The model under review builds one solid part; all positions refer to its coordinate system, in mm. Face numbers are marked on the shaded views. A direction names the side the tool comes from. Coordinates: 2 decimals unless noted, no trailing zeros. Order: outer loops, then holes, each group sorted by start corner. A loop starts at its lowest first (then second) coordinate and runs counter-clockwise, first axis right, second up.
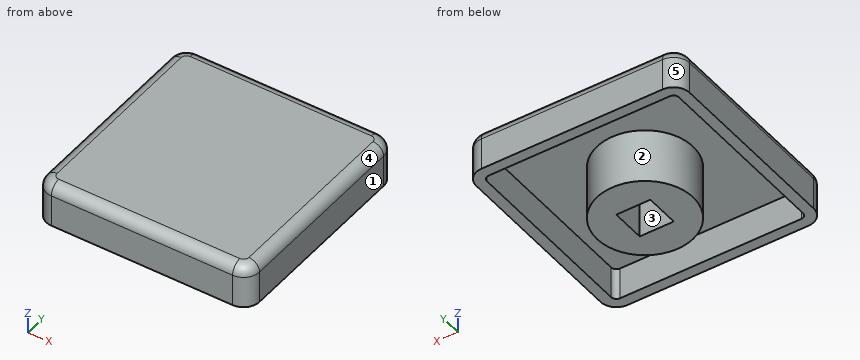
```python
from build123d import *

# Parameters (mm, degrees)
SKETCH1_R           = 4.5
SKETCH1_W           = 3.2
SKETCH1_H           = 3.2
BOSS_EXTRUDE1_DEPTH = 5.1
BOSS_EXTRUDE2_DEPTH = 1
BOSS_EXTRUDE3_START = 3
BOSS_EXTRUDE3_DEPTH = 3
FILLET1_R           = 1


with BuildPart() as part:
    # Sketch1 → Boss-Extrude1 (new body)
    with BuildSketch(Plane.XY):
        Circle(SKETCH1_R)
        Rectangle(SKETCH1_W, SKETCH1_H, mode=Mode.SUBTRACT)
    extrude(amount=BOSS_EXTRUDE1_DEPTH)

    # Sketch2 → Boss-Extrude2 (add)
    with BuildSketch(Plane.XY.offset(5.1)):
        with BuildLine():
            Line((-8.5, -10), (8.5, -10))
            ThreePointArc((8.5, -10), (9.560660172, -9.560660172), (10, -8.5))
            Line((10, -8.5), (10, 8.5))
            ThreePointArc((10, 8.5), (9.560660172, 9.560660172), (8.5, 10))
            Line((8.5, 10), (-8.5, 10))
            ThreePointArc((-8.5, 10), (-9.560660172, 9.560660172), (-10, 8.5))
            Line((-10, 8.5), (-10, -8.5))
            ThreePointArc((-10, -8.5), (-9.560660172, -9.560660172), (-8.5, -10))
        make_face()
    extrude(amount=BOSS_EXTRUDE2_DEPTH)

    # Sketch3 → Boss-Extrude3 (add)
    with BuildSketch(Plane(origin=(0, 0, 5.1), x_dir=(-1, 0, 0), z_dir=(0, 0, -1)).offset(BOSS_EXTRUDE3_START)):
        with BuildLine():
            Line((-8.5, -10), (8.5, -10))
            ThreePointArc((8.5, -10), (9.560660172, -9.560660172), (10, -8.5))
            Line((10, -8.5), (10, 8.5))
            ThreePointArc((10, 8.5), (9.560660172, 9.560660172), (8.5, 10))
            Line((8.5, 10), (-8.5, 10))
            ThreePointArc((-8.5, 10), (-9.560660172, 9.560660172), (-10, 8.5))
            Line((-10, 8.5), (-10, -8.5))
            ThreePointArc((-10, -8.5), (-9.560660172, -9.560660172), (-8.5, -10))
        make_face()
        with BuildLine():
            Line((8.5, 9), (-8.5, 9))
            ThreePointArc((-8.5, 9), (-8.853553391, 8.853553391), (-9, 8.5))
            Line((-9, 8.5), (-9, -8.5))
            ThreePointArc((-9, -8.5), (-8.853553391, -8.853553391), (-8.5, -9))
            Line((-8.5, -9), (8.5, -9))
            ThreePointArc((8.5, -9), (8.853553391, -8.853553391), (9, -8.5))
            Line((9, -8.5), (9, 8.5))
            ThreePointArc((9, 8.5), (8.853553391, 8.853553391), (8.5, 9))
        make_face(mode=Mode.SUBTRACT)
    extrude(amount=-BOSS_EXTRUDE3_DEPTH)

    # Fillet1
    fillet1_edges = [part.edges().sort_by_distance(p)[0] for p in [
        (9.560660172, -9.560660172, 6.1),
        (10, 0, 6.1),
        (9.560660172, 9.560660172, 6.1),
        (0, 10, 6.1),
        (-9.560660172, 9.560660172, 6.1),
        (-10, 0, 6.1),
        (-9.560660172, -9.560660172, 6.1),
        (0, -10, 6.1),
    ]]
    fillet(fillet1_edges, radius=FILLET1_R)


solid = part.part
```
(1) Draft analysis for pull direction Y (two halves, no side actions). For the marked faces 3, 4 and 5, state which applies: released by +Y, released by -Y, zero draft, split by the parting line, or undercut.
A:
face 3: undercut
face 4: zero draft
face 5: released by +Y
(2) Machinability: for the marked faces 1 and 2, which of the approach directions +Z, -Z, +X, -X, +Y, -Y give a long, thin tool a straight path to every point of the face, cutting with its end or side? Answer none if there is none.
A:
face 1: +Z, -Z, +X, +Y, -Y
face 2: -Z
(3) We need section B-B, the plane y = 0. Write out the cut boundary in (x, z).
A:
outline: (-10, 2.1) - (-9, 2.1) - (-9, 5.1) - (-4.5, 5.1) - (-4.5, 0) - (-1.6, 0) - (-1.6, 5.1) - (1.6, 5.1) - (1.6, 0) - (4.5, 0) - (4.5, 5.1) - (9, 5.1) - (9, 2.1) - (10, 2.1) - (10, 5.1) arc R1 ccw to (9, 6.1) - (-9, 6.1) arc R1 ccw to (-10, 5.1) - close
(4) We need section A-A, the plane z = 4.5. Write out the cut boundary in (x, y), and give its area (3 significant figures).
A:
outline: (-10, -8.5) arc R1.5 ccw to (-8.5, -10) - (8.5, -10) arc R1.5 ccw to (10, -8.5) - (10, 8.5) arc R1.5 ccw to (8.5, 10) - (-8.5, 10) arc R1.5 ccw to (-10, 8.5) - close; circle Ø9 at (0, 0); hole (-9, -8.5) arc R0.5 ccw to (-8.5, -9) - (8.5, -9) arc R0.5 ccw to (9, -8.5) - (9, 8.5) arc R0.5 ccw to (8.5, 9) - (-8.5, 9) arc R0.5 ccw to (-9, 8.5) - close; hole (-1.6, -1.6) - (1.6, -1.6) - (1.6, 1.6) - (-1.6, 1.6) - close
area: 128 mm2
(5) For pin 1 Ø1 at (x, y) = (-6.5, 8) entering from -Z; pin 2 Ø1 at (y, z) = (6, 1.5) entering from -X, all flat-tipped, find the tip position at first contact; note any pin that passes through.
A:
pin 1: stops at z = 5.1
pin 2: passes through
(6) Wall thickness on probe 1 along X at (y, z) = (-5.75, 3); probe 2 along Y at (x, z) = (-3.25, 3); probe 3 along X at (y, z) = (3.75, 4.25): over which ranges is each line inside the solid? List them lowest first.
A:
probe 1: x = -10 to -9, 9 to 10
probe 2: y = -10 to -9, -3.11 to 3.11, 9 to 10
probe 3: x = -10 to -9, -2.49 to 2.49, 9 to 10
(7) We need section D-D, the plane y = 6.5. Write out the cut boundary in (x, z).
A:
outline: (-10, 2.1) - (-9, 2.1) - (-9, 5.1) - (9, 5.1) - (9, 2.1) - (10, 2.1) - (10, 5.1) arc R1 ccw to (9, 6.1) - (-9, 6.1) arc R1 ccw to (-10, 5.1) - close
